Source: CAD feature listing. Evaluate the final solid. Frame: model axes, mm. Face numbers are marked on the shaded views. A direction names the side the tool comes from. Round coordinates to 2 decimals unless told otherwise and drop trailing zeros. Order: outer loops, then holes, each group sorted by start corner. A loop starts at its lowest first (then second) coordinate and runs counter-clockwise, first axis right, second up. Notation, with made-up numbers: (29.5, -31.5) - (67.5, -31.5) arc R28 ccw to (67.5, -2.5) - close; hole circle Ø11 at (45.5, 66). An arc over 180 degrees is marked (long way). Return JSON: item names as keys, results as strings. Group by question number.
1) Ray query, line 1 (X direction, y = -47, z = 8.5); line 2 (Y direction, x = 0, z = 0.55); line 3 (X direction, y = -15.5, z = 1.1). Return the intervals inside material, ascending. Write a range as from..to.
2) Access query for the marked faces 1, 2, 3, 4 and 5. Directions: +Z, -Z, +X, -X, +Y, -Y. A direction counts if a zero-diameter tool reaches every point of the face in a straight line with its end or side. Return the directions, or none.
3) Section A-A, the plane y = 15.5. Return loops of the section in (x, z), plus the area to 3 significant figures.
4) Section C-C, the plane y = 0. Return loops of the section in (x, z), plus the area to 3 significant figures.
5) Section B-B, the plane y = -9. Return loops of the section in (x, z).
6) Mould query, pull axis X, two halves, no side actions, for the marked faces 6, 7 and 8. Classes: pulls with the +X half, pulls with the -X half, needs draft (parallel to the pull), parting line crosses it, or undercut.
7) Section D-D, the plane x = -26. Return loops of the section in (y, z), plus the area to 3 significant figures.
8) Contact query for flat-ended pins moving along their axis: P1, Ø2, axis at y = -32.5, z = 14, coming from the +X side; P2, Ø4.5, axis at x = -15.5, y = -15.5, coming from the +Z side; P3, Ø8, axis at y = -31.5, z = 9.5, coming from the -X side; P4, Ø10, axis at x = 1.5, y = -16.5, coming from the +Z side. Output: stop coordinate, or through.
```python
from build123d import *

# Parameters (mm, degrees)
SKETCH3_R               = 11.5
SKETCH3_R_2             = 1.75
BOSS_EXTRUDE1_DEPTH     = 19
CUT_EXTRUDE1_START      = 19
SKETCH3_3_R             = 11.5
SKETCH3_3_R_2           = 1.75
CUT_EXTRUDE1_DEPTH      = 17
SKETCH3_4_R             = 1.75
SKETCH3_4_R_2           = 11.5
CUT_EXTRUDE3_DEPTH      = 38.975320933
CUT_EXTRUDE7_DEPTH      = 38.975320933
CUT_EXTRUDE7_DEPTH_BACK = 38.975320933
CUT_EXTRUDE8_DEPTH      = 38.015199581
BOSS_EXTRUDE4_DEPTH     = 19
BOSS_EXTRUDE5_START     = 19
BOSS_EXTRUDE5_DEPTH     = 3
BOSS_EXTRUDE6_DEPTH     = 6
BOSS_EXTRUDE7_START     = -6
BOSS_EXTRUDE7_DEPTH     = 16
SKETCH14_R              = 7
BOSS_EXTRUDE8_DEPTH     = 3
CUT_EXTRUDE10_DEPTH     = 13


# Read off the part's stored shape, not the designer's step: Boss-Extrude7, Cut-Extrude10
with BuildPart() as part:
    # Sketch3 → Boss-Extrude1 (new body)
    # profile 1 of 7: a face of its own
    with BuildSketch(Plane.XY):
        Polygon((-23.25, 17.798989873), (-17.798989873, 23.25), (17.798989873, 23.25), (23.25, 17.798989873), (23.25, -17.798989873), (17.798989873, -23.25), (-17.798989873, -23.25), (-23.25, -17.798989873), align=None)
        Polygon((21.25, 16.970562748), (16.970562748, 21.25), (-16.970562748, 21.25), (-21.25, 16.970562748), (-21.25, -16.970562748), (-16.970562748, -21.25), (16.970562748, -21.25), (21.25, -16.970562748), align=None, mode=Mode.SUBTRACT)
    # profile 2 of 7: a face of its own
    with BuildSketch(Plane.XY):
        Polygon((21.25, 16.970562748), (21.25, -16.970562748), (16.970562748, -21.25), (-16.970562748, -21.25), (-21.25, -16.970562748), (-21.25, 16.970562748), (-16.970562748, 21.25), (16.970562748, 21.25), align=None)
        Circle(SKETCH3_R, mode=Mode.SUBTRACT)
        with Locations((-15.5, -15.5)):
            Circle(SKETCH3_R_2, mode=Mode.SUBTRACT)
        with Locations((15.5, -15.5)):
            Circle(SKETCH3_R_2, mode=Mode.SUBTRACT)
        with Locations((15.5, 15.5)):
            Circle(SKETCH3_R_2, mode=Mode.SUBTRACT)
        with Locations((-15.5, 15.5)):
            Circle(SKETCH3_R_2, mode=Mode.SUBTRACT)
    # profile 3 of 7: a face of its own
    with BuildSketch(Plane.XY):
        with Locations((-15.5, 15.5)):
            Circle(SKETCH3_R_2)
    # profile 4 of 7: a face of its own
    with BuildSketch(Plane.XY):
        with Locations((15.5, 15.5)):
            Circle(SKETCH3_R_2)
    # profile 5 of 7: a face of its own
    with BuildSketch(Plane.XY):
        with Locations((15.5, -15.5)):
            Circle(SKETCH3_R_2)
    # profile 6 of 7: a face of its own
    with BuildSketch(Plane.XY):
        with Locations((-15.5, -15.5)):
            Circle(SKETCH3_R_2)
    # profile 7 of 7: a face of its own
    with BuildSketch(Plane.XY):
        Circle(SKETCH3_R)
    extrude(amount=BOSS_EXTRUDE1_DEPTH)

    # Sketch3<3> → Cut-Extrude1 (cut)
    with BuildSketch(Plane.XY.offset(CUT_EXTRUDE1_START)):
        Polygon((21.25, 16.970562748), (21.25, -16.970562748), (16.970562748, -21.25), (-16.970562748, -21.25), (-21.25, -16.970562748), (-21.25, 16.970562748), (-16.970562748, 21.25), (16.970562748, 21.25), align=None)
        Circle(SKETCH3_3_R, mode=Mode.SUBTRACT)
        with Locations((-15.5, -15.5)):
            Circle(SKETCH3_3_R_2, mode=Mode.SUBTRACT)
        with Locations((15.5, -15.5)):
            Circle(SKETCH3_3_R_2, mode=Mode.SUBTRACT)
        with Locations((15.5, 15.5)):
            Circle(SKETCH3_3_R_2, mode=Mode.SUBTRACT)
        with Locations((-15.5, 15.5)):
            Circle(SKETCH3_3_R_2, mode=Mode.SUBTRACT)
    extrude(amount=-CUT_EXTRUDE1_DEPTH, mode=Mode.SUBTRACT)

    # Sketch3<4> → Cut-Extrude3 (cut, through all)
    with BuildSketch(Plane.XY):
        with Locations(Location((-15.5, 15.5, 0), (0, 0, 180))):
            Circle(SKETCH3_4_R)
        with Locations(Location((15.5, 15.5, 0), (0, 0, 180))):
            Circle(SKETCH3_4_R)
        with Locations(Location((-15.5, -15.5, 0), (0, 0, 180))):
            Circle(SKETCH3_4_R)
        with Locations(Location((0, 0, 0), (0, 0, 180))):
            Circle(SKETCH3_4_R_2)
        with Locations(Location((15.5, -15.5, 0), (0, 0, 180))):
            Circle(SKETCH3_4_R)
    extrude(amount=CUT_EXTRUDE3_DEPTH, mode=Mode.SUBTRACT)

    # Sketch6 → Cut-Extrude7 (cut, two sides: drawn at the far end of the back side and taken through both)
    with BuildSketch(Plane(origin=(0, 0, 0), x_dir=(0, 0, -1), z_dir=(1, 0, 0)).offset(-CUT_EXTRUDE7_DEPTH_BACK)):
        Polygon((-19, 23.25), (-5, 23.25), (-19, -17.798989873), align=None)
    extrude(amount=CUT_EXTRUDE7_DEPTH + CUT_EXTRUDE7_DEPTH_BACK, mode=Mode.SUBTRACT)

    # Sketch8 → Cut-Extrude8 (cut, through all)
    with BuildSketch(Plane.XY.offset(2)):
        Polygon((-16.970562748, 21.25), (-14.970562748, 23.25), (14.970562748, 23.25), (16.970562748, 21.25), align=None)
    extrude(amount=CUT_EXTRUDE8_DEPTH, mode=Mode.SUBTRACT)

    # Sketch10 → Boss-Extrude4 (add)
    with BuildSketch(Plane.XY):
        Polygon((19.798989873, -21.25), (-19.798989873, -21.25), (-15.048989873, -26), (15.048989873, -26), align=None)
    extrude(amount=BOSS_EXTRUDE4_DEPTH)

    # Sketch11 → Boss-Extrude5 (add)
    with BuildSketch(Plane.XY.offset(BOSS_EXTRUDE5_START)):
        with BuildLine():
            Line((-14.556349186, -21.25), (14.556349186, -21.25))
            ThreePointArc((14.556349186, -21.25), (15.480228719, -21.867316568), (15.263455967, -22.957106781))
            Line((15.263455967, -22.957106781), (12.220562748, -26))
            Line((12.220562748, -26), (-12.220562748, -26))
            Line((-12.220562748, -26), (-15.263455967, -22.957106781))
            ThreePointArc((-15.263455967, -22.957106781), (-15.480228719, -21.867316568), (-14.556349186, -21.25))
        make_face()
    extrude(amount=BOSS_EXTRUDE5_DEPTH)


with BuildPart() as body_2:
    # Sketch12 → Boss-Extrude6 (new body)
    with BuildSketch(Plane.XY):
        with BuildLine():
            Line((2.5, -28.5), (2.5, -49.75))
            ThreePointArc((2.5, -49.75), (1.767766953, -51.517766953), (0, -52.25))
            Line((0, -52.25), (0, -57.25))
            Line((0, -57.25), (10.5, -57.25))
            Line((10.5, -57.25), (10.5, -30.548989873))
            Line((10.5, -30.548989873), (15.048989873, -26))
            Line((15.048989873, -26), (0, -26))
            ThreePointArc((0, -26), (1.767766953, -26.732233047), (2.5, -28.5))
        make_face()
    extrude(amount=BOSS_EXTRUDE6_DEPTH)

    # Boss-Extrude7 outline → Boss-Extrude7 (add)
    with BuildSketch(Plane.XY.offset(6).offset(BOSS_EXTRUDE7_START)):
        with BuildLine():
            Line((30, -61.75), (10.5, -54.5))
            Line((10.5, -54.5), (10.5, -53.982120022))
            ThreePointArc((10.5, -53.982120022), (16.833795921, -45.483677703), (7.5, -40.461651585))
            Line((7.5, -40.461651585), (7.5, -26))
            Line((7.5, -26), (0, -26))
            ThreePointArc((0, -26), (1.767766953, -26.732233047), (2.5, -28.5))
            Line((2.5, -28.5), (2.5, -49.75))
            ThreePointArc((2.5, -49.75), (1.767766953, -51.517766953), (0, -52.25))
            Line((0, -52.25), (0, -57.25))
            Line((0, -57.25), (3.562803405, -57.25))
            ThreePointArc((3.562803405, -57.25), (6.143187845, -60.341660723), (10, -61.5))
            Line((10, -61.5), (15, -61.5))
            Line((15, -61.5), (15, -64.75))
            Line((15, -64.75), (30, -64.75))
            Line((30, -64.75), (30, -61.75))
        make_face()
    extrude(amount=BOSS_EXTRUDE7_DEPTH)

    # Sketch14 → Boss-Extrude8 (add)
    with BuildSketch(Plane.XY.offset(16)):
        with Locations((10, -47)):
            Circle(SKETCH14_R)
    extrude(amount=BOSS_EXTRUDE8_DEPTH)

    # Cut-Extrude10 outline → Cut-Extrude10 (cut)
    with BuildSketch(Plane.XY):
        with BuildLine():
            ThreePointArc((12.946853826, -47.562185494), (7.188060526, -45.95453532), (12.5983656, -48.499498652))
            Line((12.5983656, -48.499498652), (16.370188856, -49.901843196))
            ThreePointArc((16.370188856, -49.901843196), (16.561192108, -49.439417579), (16.718677082, -48.964530038))
            Line((16.718677082, -48.964530038), (12.946853826, -47.562185494))
        make_face()
    extrude(amount=CUT_EXTRUDE10_DEPTH, mode=Mode.SUBTRACT)


with BuildPart() as body_3:
    # Mirror1: mirrored copy
    add(body_2.part.mirror(Plane(origin=(0, 0, 0), x_dir=(0, 0, 1), z_dir=(1, 0, 0))))


with BuildPart() as body_2_1:
    add(body_2.part)

    # Combine1: union body 3, part
    add(body_3.part)
    add(part.part)


solid = body_2_1.part
```
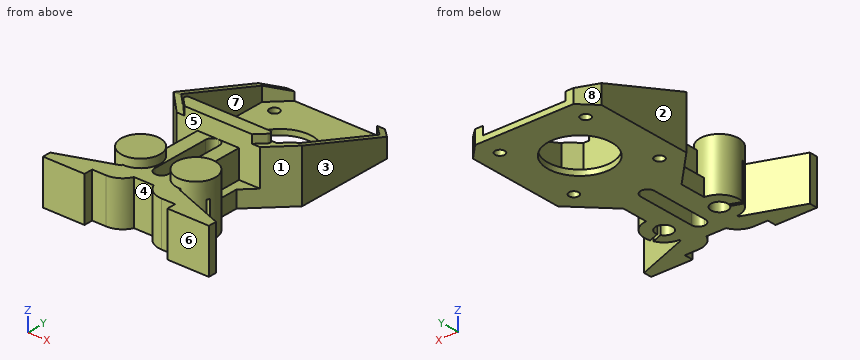
Geometry check:
{
 "1": {"line 1": "-17..-13, -7..-2.5, 2.5..7, 13..17", "line 2": "-57.25..-52.25, -26..-11.5, 11.5..23.25", "line 3": "-23.25..-17.25, -13.75..13.75, 17.25..23.25"},
 "2": {"face 1": "+Z, -Z, +X", "face 2": "+Z, -Z, -X, +Y", "face 3": "+Z, -Z, +X, +Y", "face 4": "+Z, -Z, -Y", "face 5": "+Z"},
 "3": {"outline": "(-23.25, 0) - (-17.25, 0) - (-17.25, 2) - (-21.25, 2) - (-21.25, 7.64) - (-23.25, 7.64) - close; (-13.75, 0) - (13.75, 0) - (13.75, 2) - (-13.75, 2) - close; (17.25, 0) - (23.25, 0) - (23.25, 7.64) - (21.25, 7.64) - (21.25, 2) - (17.25, 2) - close", "area": "102 mm2"},
 "4": {"outline": "(-23.25, 0) - (-11.5, 0) - (-11.5, 2) - (-21.25, 2) - (-21.25, 12.93) - (-23.25, 12.93) - close; (11.5, 0) - (23.25, 0) - (23.25, 12.93) - (21.25, 12.93) - (21.25, 2) - (11.5, 2) - close", "area": "90.7 mm2"},
 "5": {"outline": "(-23.25, 0) - (-7.16, 0) - (-7.16, 2) - (-21.25, 2) - (-21.25, 16) - (-23.25, 16) - close; (7.16, 0) - (23.25, 0) - (23.25, 16) - (21.25, 16) - (21.25, 2) - (7.16, 2) - close"},
 "6": {"face 6": "needs draft", "face 7": "undercut", "face 8": "pulls with the -X half"},
 "7": {"outline": "(-64.75, 0) - (-60.26, 0) - (-60.26, 16) - (-64.75, 16) - close", "area": "71.8 mm2"},
 "8": {"P1": "x = 7.5", "P2": "z = 2", "P3": "x = -11.49", "P4": "z = 22"}
}
